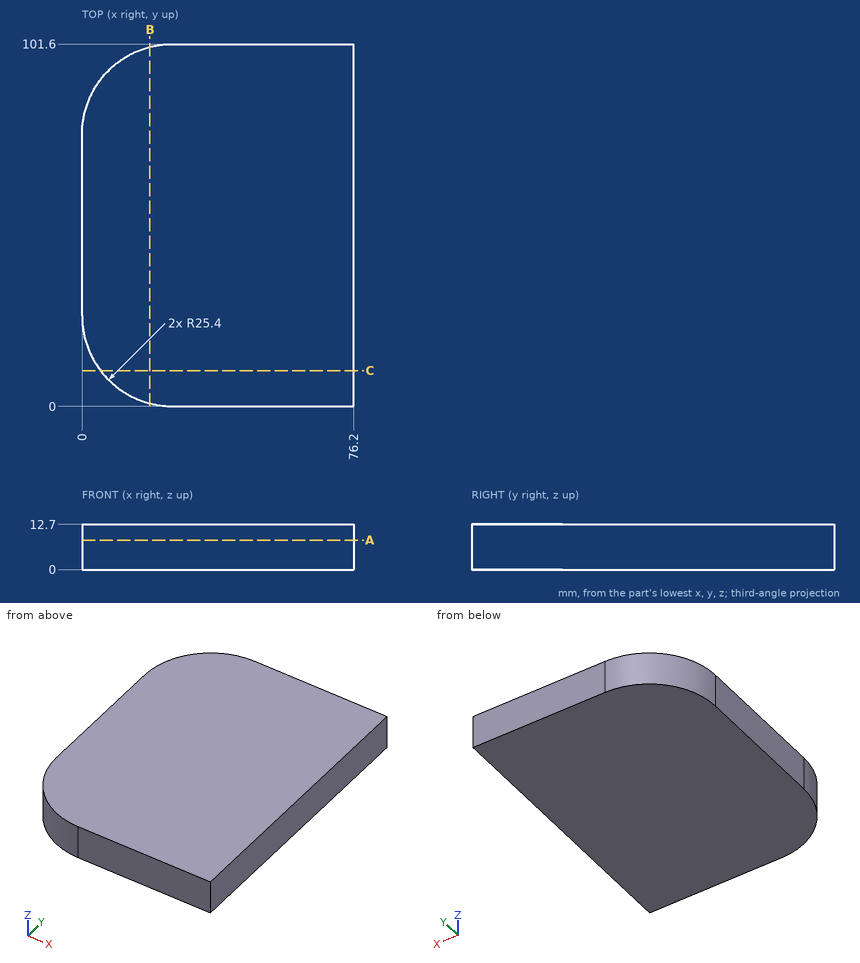
Job drawing, mm, ordinate dimensions from the low corner. One solid piece. Give positions to 0.01 mm unless a question says otherwise; leave off trailing zeros. Loops run counter-clockwise (first coordinate to the right, second up) from the corner with the lowest first, then second, coordinate; pieces in that order, holes last. Notation, with made-up numbers: (79, -29) -> (111, -29) arc R22 cw to (111, -18) -> close; hole circle Ø1 at (-4.5, -9.5). An arc over 180 degrees is marked (long way). Use a Markdown table: item, result. Add a question column.
(1) Slice it at C-C on y = 10. List the corners of the cut face in (x, z).
(2) Slice it at B-B on x = 19. List the corners of the cut face in (y, z), and give its area (3 significant figures).
(3) Slice it at A-A on z = 8.25. List the corners of the cut face in (x, y).
(4) Wall check: line 1 along Y through (x, z) = (12, 4); line 2 along X through (y, z) = (5.5, 2.75); line 3 along Y through (x, z) = (20.5, 4.5). Give the ranges that are in metal, low to high.
(5) Drop a flat-ended pin along its axis: pin 1 Ø1.5 at (y, z) = (78.5, 5.5) entering from -X. Give the stop position or say it passes through.
Filled sheet:
| question | item | result |
|---|---|---|
| 1 | outline | (5.2, 0) -> (76.2, 0) -> (76.2, 12.7) -> (5.2, 12.7) -> close |
| 2 | outline | (0.82, 0) -> (100.78, 0) -> (100.78, 12.7) -> (0.82, 12.7) -> close |
| 2 | area | 1,270 mm2 |
| 3 | outline | (0, 25.4) arc R25.4 ccw to (25.4, 0) -> (76.2, 0) -> (76.2, 101.6) -> (25.4, 101.6) arc R25.4 ccw to (0, 76.2) -> close |
| 4 | line 1 | 3.82 to 97.78 |
| 4 | line 2 | 9.62 to 76.2 |
| 4 | line 3 | 0.48 to 101.12 |
| 5 | pin 1 | x = 0.05 |
